Geometry check sheet. Reference: drawing and pictorial views, mm from the part's lowest x, y, z. A direction names the side the tool comes from. Give positions to 0.01 mm unless a question says otherwise; leave off trailing zeros. Loops run counter-clockwise (first coordinate to the right, second up) from the corner with the lowest first, then second, coordinate; pieces in that order, holes last. Notation, with made-up numbers: (78.5, -21.75) -> (106.5, -21.75) arc R11 ccw to (106.5, -17.75) -> close; hole circle Ø3 at (-8, 12.25). An arc over 180 degrees is marked (long way). One line per item, written item: value. Start each with the question number.
(1) Draft check along X on the marked faces 6, 7 and 8. Enter one of: pulls with the +X half, pulls with the -X half, needs draft (parallel to the pull), parting line crosses it, or undercut.
(2) Scan lines: line 1 along Z through (x, y) = (27, 3.9); line 2 along X through (y, z) = (30, 2.5); line 3 along X through (y, z) = (4.5, 15.25). Record each from-to range of solid material in increasing order. Write a range as from..to.
(3) Sectioned sample at B-B, the plane y = 15. Record the cut outline in (x, z), then the cut area to 3 significant figures.
(4) Sectioned sample at D-D, the plane z = 15.5. Record the cut outline in (x, y), then the cut area to 3 significant figures.
(5) Gauge pin test, flat ends, axial feed: pin 1 Ø1.3 at (x, z) = (3.5, 3) entering from -Y; pin 2 Ø1.3 at (x, z) = (4, 18) entering from +Y; pin 3 Ø10 at (x, y) = (16, 34.5) entering from +Z. Record the tip position at first contact, or that the pin passes through.
(6) Sectioned sample at A-A, the plane z = 18. Record the cut outline in (x, y), then the cut area to 3 significant figures.
(7) Sectioned sample at C-C, the plane x = 27. Record the cut outline in (y, z), then the cut area to 3 significant figures.
(8) Tool access check on the marked faces 1, 2, 3, 4 and 5. Record the directions out of +Z, -Z, +X, -X, +Y, -Y that give a thin tool (end or side, any length) a straight path to the whole face; none if there is none.
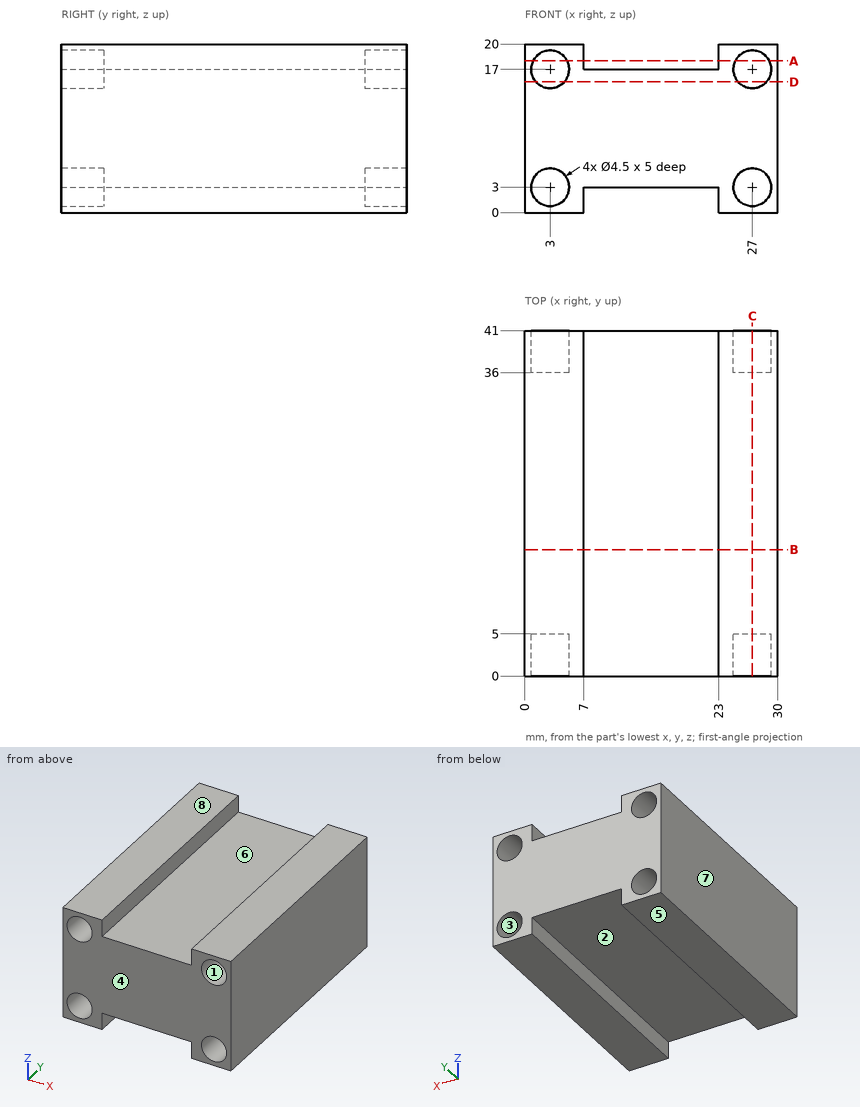
Calculated:
1. face 6: undercut
1. face 7: pulls with the -X half
1. face 8: needs draft
2. line 1: z = 0..0.75, 5.25..14.75, 19.25..20
2. line 2: x = 0..7, 23..30
2. line 3: x = 0..1.59, 4.41..25.59, 28.41..30
3. outline: (0, 0) -> (7, 0) -> (7, 3) -> (23, 3) -> (23, 0) -> (30, 0) -> (30, 20) -> (23, 20) -> (23, 17) -> (7, 17) -> (7, 20) -> (0, 20) -> close
3. area: 504 mm2
4. outline: (0, 0) -> (1.32, 0) -> (1.32, 5) -> (4.68, 5) -> (4.68, 0) -> (25.32, 0) -> (25.32, 5) -> (28.68, 5) -> (28.68, 0) -> (30, 0) -> (30, 41) -> (28.68, 41) -> (28.68, 36) -> (25.32, 36) -> (25.32, 41) -> (4.68, 41) -> (4.68, 36) -> (1.32, 36) -> (1.32, 41) -> (0, 41) -> close
4. area: 1,160 mm2
5. pin 1: stops at y = 5
5. pin 2: stops at y = 36
5. pin 3: stops at z = 17
6. outline: (0, 0) -> (0.98, 0) -> (0.98, 5) -> (5.02, 5) -> (5.02, 0) -> (7, 0) -> (7, 41) -> (5.02, 41) -> (5.02, 36) -> (0.98, 36) -> (0.98, 41) -> (0, 41) -> close; (23, 0) -> (24.98, 0) -> (24.98, 5) -> (29.02, 5) -> (29.02, 0) -> (30, 0) -> (30, 41) -> (29.02, 41) -> (29.02, 36) -> (24.98, 36) -> (24.98, 41) -> (23, 41) -> close
6. area: 493 mm2
7. outline: (0, 0) -> (41, 0) -> (41, 0.75) -> (36, 0.75) -> (36, 5.25) -> (41, 5.25) -> (41, 14.75) -> (36, 14.75) -> (36, 19.25) -> (41, 19.25) -> (41, 20) -> (0, 20) -> (0, 19.25) -> (5, 19.25) -> (5, 14.75) -> (0, 14.75) -> (0, 5.25) -> (5, 5.25) -> (5, 0.75) -> (0, 0.75) -> close
7. area: 730 mm2
8. face 1: -Y
8. face 2: -Z, +Y, -Y
8. face 3: +Y
8. face 4: +Z, -Z, +X, -X, -Y
8. face 5: -Z, +X, -X, +Y, -Y
